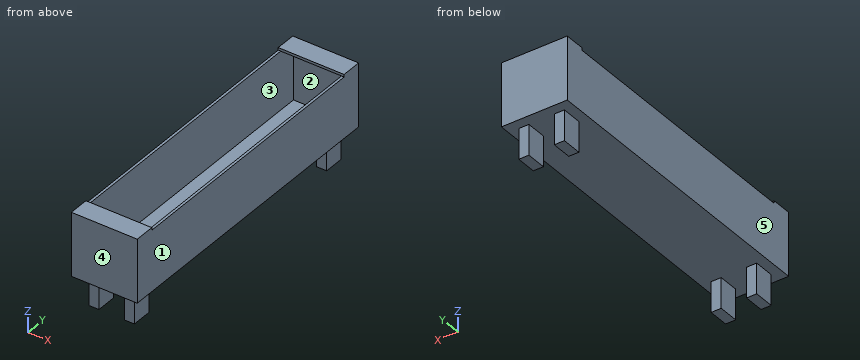
from build123d import *

# Parameters (mm, degrees)
F0_W     = 304.8
F0_H     = 12.7
F1_DEPTH = 1524
F3_DEPTH = 1524
F4_W     = 12.7
F4_H     = 304.8
F5_DEPTH = 330.2
F6_W     = 101.6
F6_H     = 12.7
F7_DEPTH = 330.2
F8_W     = 50.8
F8_H     = 101.6
F9_DEPTH = 152.4


with BuildPart() as f1:
    # F0 (on Front) → F1 (new body)
    with BuildSketch(Plane.XZ):
        with Locations((-108.432242626, -17.0491518617)):
            Rectangle(F0_W, F0_H)
    extrude(amount=F1_DEPTH)

    # F2 (on face) → F3 (join)
    with BuildSketch(Plane.XZ.offset(1524)):
        Polygon((-273.532242626, -23.3991518617), (-260.832242626, -23.3991518617), (-260.832242626, -10.6991518617), (-260.832242626, 281.4008481383), (-273.532242626, 281.4008481383), align=None)
        Polygon((43.967757374, -10.6991518617), (43.967757374, -23.3991518617), (56.667757374, -23.3991518617), (56.667757374, 281.4008481383), (43.967757374, 281.4008481383), align=None)
    extrude(amount=-F3_DEPTH)

    # F4 (on face) → F5 (join)
    with BuildSketch(Plane(origin=(-273.532242626, 0, 0), x_dir=(0, -1, 0), z_dir=(-1, 0, 0))):
        with Locations((-6.35, 129.0008481383)):
            Rectangle(F4_W, F4_H)
        with Locations((1530.35, 129.0008481383)):
            Rectangle(F4_W, F4_H)
    extrude(amount=-F5_DEPTH)

    # F6 (on face) → F7 (join)
    with BuildSketch(Plane(origin=(-273.532242626, 0, 0), x_dir=(0, -1, 0), z_dir=(-1, 0, 0))):
        with Locations((1485.9, 287.7508481383)):
            Rectangle(F6_W, F6_H)
        with Locations((38.1, 287.7508481383)):
            Rectangle(F6_W, F6_H)
    extrude(amount=-F7_DEPTH)

    # F8 (on face) → F9 (join)
    with BuildSketch(Plane(origin=(0, 0, -23.3991518617), x_dir=(1, 0, 0), z_dir=(0, 0, -1))):
        with Locations((-197.332242626, 88.9)):
            Rectangle(F8_W, F8_H)
        with Locations((-19.532242626, 88.9)):
            Rectangle(F8_W, F8_H)
        with Locations((-197.332242626, 1435.1)):
            Rectangle(F8_W, F8_H)
        with Locations((-19.532242626, 1435.1)):
            Rectangle(F8_W, F8_H)
    extrude(amount=F9_DEPTH)


solid = f1.part
Design review of the part built by this model. Coordinates are the model's own, in mm. Face numbers are marked on the shaded views. A direction names the side the tool comes from. Give positions to 0.01 mm unless a question says otherwise; leave off trailing zeros. Loops run counter-clockwise (first coordinate to the right, second up) from the corner with the lowest first, then second, coordinate; pieces in that order, holes last. Notation, with made-up numbers: M -21.75,52 L 20.25,52 A15 cw 20.25,72 Z; hole C -16.75,31 d8. An arc over 180 degrees is marked long. Write item = value, one per line.
Q1. We need section B-B (y = -1145.5). Give the boundary of the cut face in (x, z).
Output values:
outline = M -273.53,-23.4 L 56.67,-23.4 L 56.67,281.4 L 43.97,281.4 L 43.97,-10.7 L -260.83,-10.7 L -260.83,281.4 L -273.53,281.4 Z
Q2. We need section C-C (x = -111.5). Give the boundary of the cut face in (y, z), plus the area to 3 significant figures.
Output values:
outline = M -1536.7,-23.4 L 12.7,-23.4 L 12.7,294.1 L -88.9,294.1 L -88.9,281.4 L 0,281.4 L 0,-10.7 L -1524,-10.7 L -1524,281.4 L -1435.1,281.4 L -1435.1,294.1 L -1536.7,294.1 Z
area = 29,700 mm^2
Q3. We need section D-D (x = -7.5). Give the boundary of the cut face in (y, z), plus the area to 3 significant figures.
Output values:
outline = M -1536.7,-23.4 L -1485.9,-23.4 L -1485.9,-175.8 L -1384.3,-175.8 L -1384.3,-23.4 L -139.7,-23.4 L -139.7,-175.8 L -38.1,-175.8 L -38.1,-23.4 L 12.7,-23.4 L 12.7,294.1 L -88.9,294.1 L -88.9,281.4 L 0,281.4 L 0,-10.7 L -1524,-10.7 L -1524,281.4 L -1435.1,281.4 L -1435.1,294.1 L -1536.7,294.1 Z
area = 60,600 mm^2
Q4. To check wall thickness, follow line 1 (X direction, y = -556.5, z = 206); line 2 (Y direction, x = -56.5, z = 175.5); line 3 (Z direction, x = -191, y = -579.5). State the ranges of each line that lie inside material, in increasing order. Write a range as [from, to].
Output values:
line_1 = [-273.53, -260.83], [43.97, 56.67]
line_2 = [-1536.7, -1524], [0, 12.7]
line_3 = [-23.4, -10.7]
Q5. We need section A-A (z = 217). Give the boundary of the cut face in (x, y).
Output values:
outline = M -273.53,-1536.7 L 56.67,-1536.7 L 56.67,12.7 L -273.53,12.7 Z; hole M -260.83,-1524 L 43.97,-1524 L 43.97,0 L -260.83,0 Z
Q6. Insertion check: pin 1 (10 mm diameter, centred on x = -71.5, y = -611.5, fed in from -Z); pin 2 (14 mm diameter, centred on x = -266, y = -446, fed in from +Z). Each pin has a flat end and moves straight along its axis. Give the tip position at first contact, or say it passes through.
Output values:
pin_1 = -23.4
pin_2 = 281.4
Q7. Draft analysis for pull direction Y (two halves, no side actions). For the marked faces 3, 4 and 5, state which applies: +Y half, -Y half, draft (parallel to the pull), parting line (faces both ways), or undercut.
Output values:
face_3 = undercut
face_4 = -Y half
face_5 = draft
Q8. For the marked faces 1 and 2, list the 3-axis set-ups (+Z, -Z, +X, -X, +Y, -Y) from which the entire face can be reached by the end or side of a thin tool; tool diameter is ignored.
Output values:
face_1 = +Z, -Z, +X, +Y, -Y
face_2 = none
